from build123d import *

# Parameters (mm, degrees)
F0_W     = 33.8836
F0_H     = 71.755
F1_DEPTH = 2.54
F2_W     = 6.35
F2_H     = 71.755
F3_DEPTH = 8.89
F4_R     = 2.159
F5_DEPTH = 6.35


with BuildPart() as f1:
    # F0 (on Top) → F1 (new body)
    with BuildSketch(Plane.XY):
        with Locations((-16.9418, 1.956956)):
            Rectangle(F0_W, F0_H)
    extrude(amount=F1_DEPTH)

    # F2 (on face) → F3 (join)
    with BuildSketch(Plane.XY.offset(2.54)):
        with Locations((-16.9418, 1.956956)):
            Rectangle(F2_W, F2_H)
    extrude(amount=F3_DEPTH)

    # F4 (on face) → F5 (cut)
    with BuildSketch(Plane(origin=(-20.1168, 0, 0), x_dir=(0, -1, 0), z_dir=(-1, 0, 0))):
        with Locations((-18.212956, 6.858)):
            Circle(F4_R)
        with Locations((-34.468956, 6.858)):
            Circle(F4_R)
        with Locations((-1.956956, 6.858)):
            Circle(F4_R)
        with Locations((14.299044, 6.858)):
            Circle(F4_R)
        with Locations((30.555044, 6.858)):
            Circle(F4_R)
    extrude(amount=-F5_DEPTH, mode=Mode.SUBTRACT)


solid = f1.part
Read the model definition and answer for the solid it produces. Units are mm, in the model's axes. A direction names the side the tool comes from. Round coordinates to 2 decimals unless told otherwise and drop trailing zeros. Order: outer loops, then holes, each group sorted by start corner. A loop starts at its lowest first (then second) coordinate and runs counter-clockwise, first axis right, second up.
1) The mould has two halves that part along Z. Classify faces 1 (the face through (-17, 2, 0)), 2 (the face through (-16.99, 16.22, 6.03)), 3 (the face through (-17, 2, 11.43)): released by +Z, released by -Z, zero draft, split by the parting line, or undercut.
2) The part is cut by section B-B on z = 7.5. Write down the section's boundary in (x, y).
3) For faces 4 (the face through (-20.117, 1, 10)), 5 (the face through (-13.767, 1, 10)), 6 (the face through (-33.884, 1, 1)), determine the directions among +Z, -Z, +X, -X, +Y, -Y from which every point of the face is accessible in a straight line to the end or side of a thin tool.
4) Flat-ended cylindrical pins translate along their axes: pin 1 (7 mm diameter, centred on x = -6.5, y = 0, fed in from +Z); pin 2 (12 mm diameter, centred on x = -11, y = 19.5, fed in from +Z); pin 3 (4 mm diameter, centred on y = 4.5, z = 9.5, fed in from -X). Find the tip coordinate at first contact, or state that the pin passes through.
5) Straight lines are drawn through the part: L1, parallel to Z at x = -25, y = 12.5; L2, parallel to Z at x = -16, y = 19; L3, parallel to X at y = -10.5, z = 9.5. For each, find the intervals that lie inside material, in ascending order.
6) The part is cut by section A-A on y = -13.5. Write down the section's boundary in (x, z).
7) The part is cut by section C-C on x = -15.5. Write down the section's boundary in (y, z), plus the area to 3 significant figures.
8) The part is cut by section D-D on y = -27.5. Write down the section's boundary in (x, z), plus the area to 3 significant figures.
Resolved:
1. face 1: released by -Z
1. face 2: undercut
1. face 3: released by +Z
2. outline: (-20.12, -33.92) - (-13.77, -33.92) - (-13.77, -32.62) - (-20.12, -32.62) - close; (-20.12, -28.49) - (-13.77, -28.49) - (-13.77, -16.36) - (-20.12, -16.36) - close; (-20.12, -12.24) - (-13.77, -12.24) - (-13.77, -0.1) - (-20.12, -0.1) - close; (-20.12, 4.02) - (-13.77, 4.02) - (-13.77, 16.15) - (-20.12, 16.15) - close; (-20.12, 20.27) - (-13.77, 20.27) - (-13.77, 32.41) - (-20.12, 32.41) - close; (-20.12, 36.53) - (-13.77, 36.53) - (-13.77, 37.83) - (-20.12, 37.83) - close
3. face 4: +Z, -X, +Y, -Y
3. face 5: +Z, +X, +Y, -Y
3. face 6: +Z, -Z, -X, +Y, -Y
4. pin 1: stops at z = 2.54
4. pin 2: stops at z = 11.43
4. pin 3: stops at x = -20.12
5. L1: z = 0 to 2.54
5. L2: z = 0 to 4.85, 8.87 to 11.43
5. L3: x = -20.12 to -13.77
6. outline: (-33.88, 0) - (0, 0) - (0, 2.54) - (-13.77, 2.54) - (-13.77, 4.85) - (-20.12, 4.85) - (-20.12, 2.54) - (-33.88, 2.54) - close; (-20.12, 8.86) - (-13.77, 8.86) - (-13.77, 11.43) - (-20.12, 11.43) - close
7. outline: (-33.92, 0) - (37.83, 0) - (37.83, 11.43) - (-33.92, 11.43) - close; hole circle Ø4.32 at (-30.56, 6.86); hole circle Ø4.32 at (-14.3, 6.86); hole circle Ø4.32 at (1.96, 6.86); hole circle Ø4.32 at (18.21, 6.86); hole circle Ø4.32 at (34.47, 6.86)
7. area: 747 mm2
8. outline: (-33.88, 0) - (0, 0) - (0, 2.54) - (-13.77, 2.54) - (-13.77, 11.43) - (-20.12, 11.43) - (-20.12, 2.54) - (-33.88, 2.54) - close
8. area: 143 mm2
